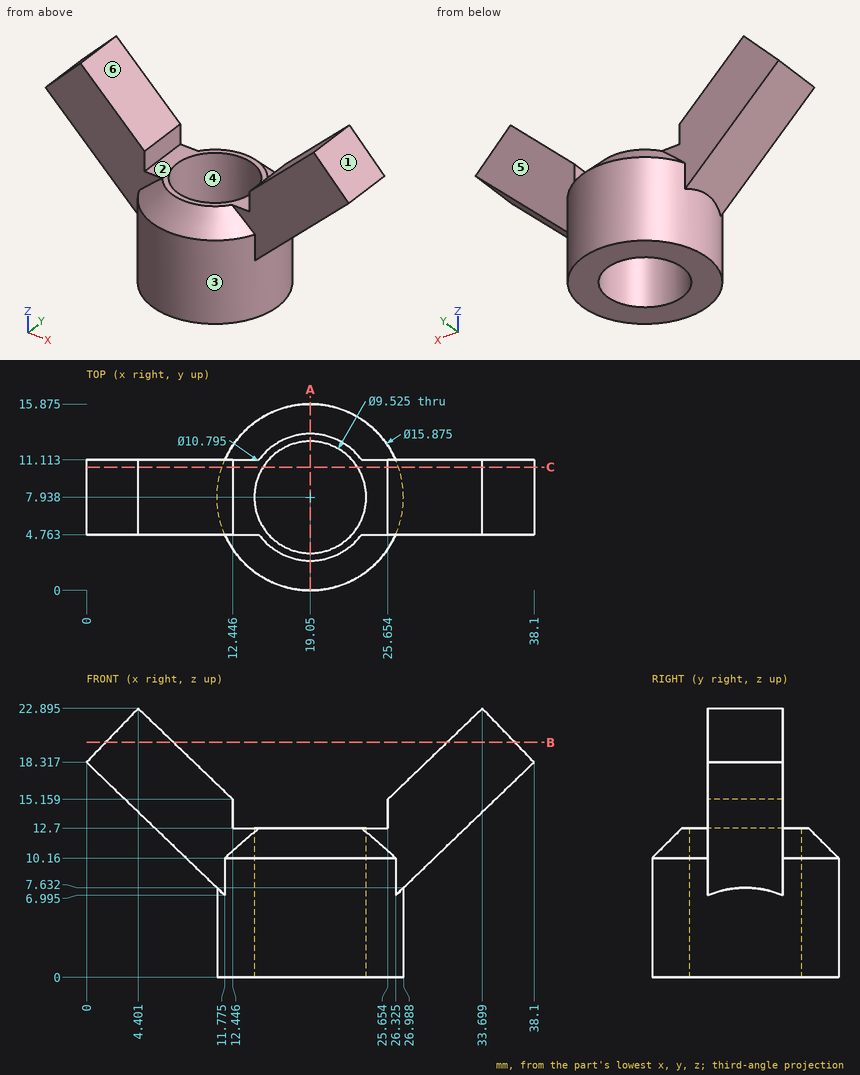
Can you work these out from the drawing? Everything is in mm from the part's minimum corner. A direction names the side the tool comes from. Round coordinates to 2 decimals unless told otherwise and drop trailing zeros. Loops run counter-clockwise (first coordinate to the right, second up) from the corner with the lowest first, then second, coordinate; pieces in that order, holes last. Notation, with made-up numbers: (-31, 13) -> (-10, 13) arc R23 cw to (-10, 48) -> close; hole circle Ø7 at (51.5, -28.75). An arc over 180 degrees is marked (long way). Answer in a Markdown table with one row per item.
Item 1: We'd pull the mould along Y, two halves only. Please class the marked faces 4, 5 and 6: released by +Y, released by -Y, zero draft, split by the parting line, or undercut.
Answer block:
| item | result |
|---|---|
| face 4 | undercut |
| face 5 | released by +Y |
| face 6 | zero draft |
Item 2: If I drill on probe 1 along Y at (x, z) = (19.05, 5) (1 decimal); probe 2 along X at (y, z) = (11, 11) (1 decimal); probe 3 along X at (y, z) = (7, 18.5) (1 decimal), over which ranges is the centre line in solid material (lowest first)?
Answer block:
| item | result |
|---|---|
| probe 1 | 0 to 3.2, 12.7 to 15.9 |
| probe 2 | 7.6 to 15.4, 22.7 to 30.5 |
| probe 3 | 0.2 to 9, 29.1 to 37.9 |
Item 3: On a 3-axis mill with a long thin cutter (end or side, diameter ignored), from which of +Z, -Z, +X, -X, +Y, -Y can I reach the whole of each face in a straight line? I mean the marked faces 1, 2 and 3. Say none if no direction works.
Answer block:
| item | result |
|---|---|
| face 1 | +Z, +X, +Y, -Y |
| face 2 | +Z, +Y, -Y |
| face 3 | -Z |
Item 4: Suppose I cut it at A-A, the plane x = 19.05. List the corners of the cut face in (y, z) for me (1 decimal).
Answer block:
| item | result |
|---|---|
| outline | (0, 0) -> (3.2, 0) -> (3.2, 12.7) -> (2.5, 12.7) -> (0, 10.2) -> close; (12.7, 0) -> (15.9, 0) -> (15.9, 10.2) -> (13.3, 12.7) -> (12.7, 12.7) -> close |
Item 5: Suppose I cut it at C-C, the plane y = 10.5. List the corners of the cut face in (x, z) for me (1 decimal).
Answer block:
| item | result |
|---|---|
| outline | (0, 18.3) -> (11.5, 7.2) -> (11.5, 0) -> (15, 0) -> (15, 12.7) -> (12.4, 12.7) -> (12.4, 15.2) -> (4.4, 22.9) -> close; (23.1, 0) -> (26.6, 0) -> (26.6, 7.2) -> (38.1, 18.3) -> (33.7, 22.9) -> (25.7, 15.2) -> (25.7, 12.7) -> (23.1, 12.7) -> close |
Item 6: Suppose I cut it at B-B, the plane z = 20. List the corners of the cut face in (x, y) for me.
Answer block:
| item | result |
|---|---|
| outline | (1.62, 4.76) -> (7.41, 4.76) -> (7.41, 11.11) -> (1.62, 11.11) -> close; (30.69, 4.76) -> (36.48, 4.76) -> (36.48, 11.11) -> (30.69, 11.11) -> close |
Item 7: Will these pins go through, and if not, where does the flat tip stop? P1, Ø12, axis at x = 28, z = 6, coming from the +Y side; P2, Ø7.5, axis at x = 32, z = 13, coming from the +Y side; P3, Ø8, axis at y = 14, z = 14.5, coming from the +X side.
Answer block:
| item | result |
|---|---|
| P1 | y = 15.31 |
| P2 | y = 11.11 |
| P3 | x = 37.01 |
